from build123d import *

# Parameters (mm, degrees)
ESQUISSE1_W                  = 26
ESQUISSE1_H                  = 48
BOSS_EXTRU_1_DEPTH           = 3
ESQUISSE2_R                  = 2
ENL_V_MAT_EXTRU_1_DEPTH      = 1
ENL_V_MAT_EXTRU_1_DEPTH_BACK = 4
ESQUISSE3_R                  = 2.25
ENL_V_MAT_EXTRU_2_DEPTH      = 1
ENL_V_MAT_EXTRU_2_DEPTH_BACK = 4
ESQUISSE4_R                  = 2.5
ENL_V_MAT_EXTRU_3_DEPTH      = 0.4
CONG_1_R                     = 2


with BuildPart() as part:
    # Esquisse1 → Boss.-Extru.1 (new body)
    with BuildSketch(Plane.XY):
        with Locations((13, 24)):
            Rectangle(ESQUISSE1_W, ESQUISSE1_H)
    extrude(amount=BOSS_EXTRU_1_DEPTH)

    # Esquisse2 → Enlèv. mat.-Extru.1 (cut, two sides)
    with BuildSketch(Plane.XY.offset(3)) as enl_v_mat_extru_1_sk:
        with Locations((4, 44)):
            Circle(ESQUISSE2_R)
        with Locations((4, 32)):
            Circle(ESQUISSE2_R)
        with Locations((22, 32)):
            Circle(ESQUISSE2_R)
        with Locations((22, 44)):
            Circle(ESQUISSE2_R)
    extrude(amount=ENL_V_MAT_EXTRU_1_DEPTH, mode=Mode.SUBTRACT)
    extrude(enl_v_mat_extru_1_sk.sketch, amount=-ENL_V_MAT_EXTRU_1_DEPTH_BACK, mode=Mode.SUBTRACT)

    # Esquisse3 → Enlèv. mat.-Extru.2 (cut, two sides)
    with BuildSketch(Plane.XY.offset(3)) as enl_v_mat_extru_2_sk:
        with Locations((13, 5)):
            Circle(ESQUISSE3_R)
        with Locations((4, 5)):
            Circle(ESQUISSE3_R)
        with Locations((22, 5)):
            Circle(ESQUISSE3_R)
    extrude(amount=ENL_V_MAT_EXTRU_2_DEPTH, mode=Mode.SUBTRACT)
    extrude(enl_v_mat_extru_2_sk.sketch, amount=-ENL_V_MAT_EXTRU_2_DEPTH_BACK, mode=Mode.SUBTRACT)

    # Esquisse4 → Enlèv. mat.-Extru.3 (cut)
    with BuildSketch(Plane.XY.offset(3)):
        with Locations((4, 32)):
            Circle(ESQUISSE4_R)
        with Locations((22, 32)):
            Circle(ESQUISSE4_R)
        with Locations((22, 44)):
            Circle(ESQUISSE4_R)
        with Locations((4, 44)):
            Circle(ESQUISSE4_R)
    extrude(amount=-ENL_V_MAT_EXTRU_3_DEPTH, mode=Mode.SUBTRACT)

    # Congé1
    cong_1_edges = [part.edges().sort_by_distance(p)[0] for p in [
        (0, 48, 1.5),
        (26, 48, 1.5),
        (26, 0, 1.5),
        (0, 0, 1.5),
    ]]
    fillet(cong_1_edges, radius=CONG_1_R)


solid = part.part
CAD build for the part. Positions are in the model's coordinates, mm. A direction names the side the tool comes from. Give positions to 0.01 mm unless a question says otherwise; leave off trailing zeros. Write each loop counter-clockwise with the first axis right and the second up, starting at its lowest first coordinate (ties: lowest second). Pieces come first, ordered by that corner, then holes. Notation, with made-up numbers: (-0.5, -22.5) -> (42.5, -22.5) arc R19 cw to (42.5, -8.5) -> close; hole circle Ø5 at (-24.5, -21.75). An arc over 180 degrees is marked (long way). Return JSON: item names as keys, results as strings.
Item 1: Two-plate mould, pull along Y, no slides. Class faces 1 (the flat face through (13, 24, 0)), 2 (the cylindrical face through (0.57, 47.4, 1.52)), 3 (the cylindrical face through (4, 30, 1)): +Y half, -Y half, draft (parallel to the pull), parting line (faces both ways), or undercut.
Answer below:
{"face 1": "draft", "face 2": "+Y half", "face 3": "undercut"}
Item 2: Drill centre lines: probe 1 along Y at (x, z) = (4, 2.8); probe 2 along Y at (x, z) = (4, 0.6); probe 3 along X at (y, z) = (31, 2.9). Where is each one in solid material? Low to high.
Answer below:
{"probe 1": "y = 0 to 2.75, 7.25 to 29.5, 34.5 to 41.5, 46.5 to 48", "probe 2": "y = 0 to 2.75, 7.25 to 30, 34 to 42, 46 to 48", "probe 3": "x = 0 to 1.71, 6.29 to 19.71, 24.29 to 26"}
Item 3: Band-saw the part on B-B (x = 22). List the corners of the cut face in (y, z), then the cut area to 3 significant figures.
Answer below:
{"outline": "(0, 0) -> (2.75, 0) -> (2.75, 3) -> (0, 3) -> close; (7.25, 0) -> (30, 0) -> (30, 2.6) -> (29.5, 2.6) -> (29.5, 3) -> (7.25, 3) -> close; (34, 0) -> (42, 0) -> (42, 2.6) -> (41.5, 2.6) -> (41.5, 3) -> (34.5, 3) -> (34.5, 2.6) -> (34, 2.6) -> close; (46, 0) -> (48, 0) -> (48, 3) -> (46.5, 3) -> (46.5, 2.6) -> (46, 2.6) -> close", "area": "106 mm2"}
Item 4: Tool access for faces 4 (the cylindrical face through (22, 30, 1)), 5 (the cylindrical face through (20, 42.5, 2.8)): list every direction of +Z, -Z, +X, -X, +Y, -Y with a clear straight run to the whole face (end or side of a thin tool).
Answer below:
{"face 4": "+Z, -Z", "face 5": "+Z"}
Item 5: Drop a flat-ended pin along its axis: pin 1 (4.5 mm diameter, centred on x = 22, y = 32, fed in from +Z). Give the stop position or say it passes through.
Answer below:
{"pin 1": "stops at z = 2.6"}
Item 6: Band-saw the part on C-C (y = 44). List the corners of the cut face in (x, z).
Answer below:
{"outline": "(0, 0) -> (2, 0) -> (2, 2.6) -> (1.5, 2.6) -> (1.5, 3) -> (0, 3) -> close; (6, 0) -> (20, 0) -> (20, 2.6) -> (19.5, 2.6) -> (19.5, 3) -> (6.5, 3) -> (6.5, 2.6) -> (6, 2.6) -> close; (24, 0) -> (26, 0) -> (26, 3) -> (24.5, 3) -> (24.5, 2.6) -> (24, 2.6) -> close"}
Item 7: Band-saw the part on D-D (z = 0.55). List the corners of the cut face in (x, y).
Answer below:
{"outline": "(0, 2) arc R2 ccw to (2, 0) -> (24, 0) arc R2 ccw to (26, 2) -> (26, 46) arc R2 ccw to (24, 48) -> (2, 48) arc R2 ccw to (0, 46) -> close; hole circle Ø4.5 at (4, 5); hole circle Ø4 at (4, 32); hole circle Ø4 at (4, 44); hole circle Ø4.5 at (13, 5); hole circle Ø4.5 at (22, 5); hole circle Ø4 at (22, 32); hole circle Ø4 at (22, 44)"}
Item 8: Band-saw the part on A-A (y = 5). List the corners of the cut face in (x, z).
Answer below:
{"outline": "(0, 0) -> (1.75, 0) -> (1.75, 3) -> (0, 3) -> close; (6.25, 0) -> (10.75, 0) -> (10.75, 3) -> (6.25, 3) -> close; (15.25, 0) -> (19.75, 0) -> (19.75, 3) -> (15.25, 3) -> close; (24.25, 0) -> (26, 0) -> (26, 3) -> (24.25, 3) -> close"}
